Autodesk Inventor part; units mm, degrees
ref_plane "YZ Plane" through (0, 0, 0) normal (1, 0, 0) x (0, 1, 0)
ref_plane "XZ Plane" through (0, 0, 0) normal (0, 1, 0) x (-1, 0, 0)
ref_plane "XY Plane" through (0, 0, 0) normal (0, 0, 1) x (1, 0, 0)
sketch "スケッチ1" plane through (0, 0, 0) normal (1, 0, 0) x (0, 1, 0)
  circle A0 centre (0, 0) radius 4
  dimension "d0" = 8
extrude "押し出し1" add sketch "スケッチ1" along normal blind 25.5
sketch "スケッチ2" plane through (25.5, 0, 0) normal (1, 0, 0) x (0, 0, -1)
  circle A0 centre (0, 0) radius 6
  circle A1 centre (0, 0) radius 4
  dimension "d3" = 12
extrude "押し出し2" add sketch "スケッチ2" against normal blind 2.9
sketch "スケッチ3" plane through (22.6, 0, 0) normal (-1, 0, 0) x (0, 0, 1)
  circle A0 centre (0, 0) radius 3.6421
  circle A1 centre (-0.1483, 0) radius 6.8
  dimension "d6" = 13.6
extrude "押し出し3" add sketch "スケッチ3" along normal blind 2.6
sketch "スケッチ4" plane through (20, 0, -0.1483) normal (-1, 0, 0) x (0, 0, 1)
  circle A0 centre (0.1483, 0) radius 4
  circle A1 centre (0.1483, 0) radius 6
extrude "押し出し4" add sketch "スケッチ4" along normal blind 2.9
sketch "スケッチ5" plane through (25.5, 0, 0) normal (1, 0, 0) x (0, 0, -1)
  circle A0 centre (0, 0) radius 3
  dimension "d11" = 6
extrude "押し出し5" cut sketch "スケッチ5" against normal blind 1
properties part number "encoderaxis"
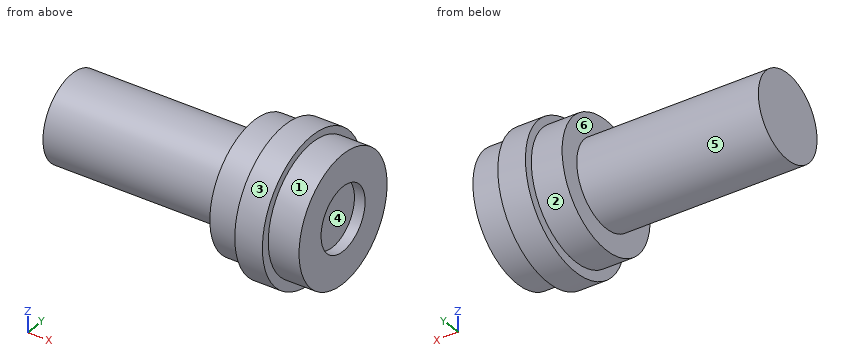
Read the model definition and answer for the solid it produces. Units are mm, in the model's axes. Face numbers are marked on the shaded views. A direction names the side the tool comes from. Give positions to 0.01 mm unless a question says otherwise; leave off trailing zeros. Write each loop counter-clockwise with the first axis right and the second up, starting at its lowest first coordinate (ties: lowest second). Pieces come first, ordered by that corner, then holes. Notation, with made-up numbers: (12.5, 8.25) - (70.5, 8.25) arc R17 cw to (70.5, 15.25) - close; hole circle Ø9 at (15, -38). An arc over 180 degrees is marked (long way). Use CSV: the item, a comma, the result in double quotes. Start each with the question number.
(1) Find section C-C (z = 0). Give the vertices of the cut face in (x, y), plus the area to 3 significant figures.
(2) Find section B-B (x = 19.5). Give the vertices of the cut face in (y, z).
(3) Determine the mould class of the marked faces 4, 5 and 6 for opening direction Y: +Y half, -Y half, draft (parallel to the pull), parting line (faces both ways), or undercut.
(4) Find section D-D (y = 5.25). Give the vertices of the cut face in (x, z).
(5) Consider line 1 along Y through (x, z) = (24.8, 0); line 2 along X through (y, z) = (-4.5, 0); line 3 along X through (y, z) = (-5, -3.5). Determine where each line is inside the solid, lowest interval first.
(6) Given P1, Ø2, axis at x = 22.5, y = -5, coming from the -Z side; P2, Ø1, axis at x = 22.5, y = 2.5, coming from the -Z side; P3, Ø1.8, axis at y = -1.5, z = 0, coming from the +X side, each flat-ended and moving along its own axis, determine where each tip first touches the part or whether it passes through.
(7) Find section A-A (y = 0). Give the vertices of the cut face in (x, z).
(8) For the marked faces 1, 2 and 3, determine the directions among +Z, -Z, +X, -X, +Y, -Y from which every point of the face is accessible in a straight line to the end or side of a thin tool.
Findings below:
1,outline,"(0, -4) - (17.1, -4) - (17.1, -6) - (20, -6) - (20, -6.8) - (22.6, -6.8) - (22.6, -6) - (25.5, -6) - (25.5, -3) - (24.5, -3) - (24.5, 3) - (25.5, 3) - (25.5, 6) - (22.6, 6) - (22.6, 6.8) - (20, 6.8) - (20, 6) - (17.1, 6) - (17.1, 4) - (0, 4) - close"
1,area,"236 mm2"
2,outline,"circle Ø12 at (0, 0)"
3,face 4,"undercut"
3,face 5,"parting line"
3,face 6,"draft"
4,outline,"(17.1, -2.9) - (20, -2.9) - (20, -4.47) - (22.6, -4.47) - (22.6, -2.9) - (25.5, -2.9) - (25.5, 2.9) - (22.6, 2.9) - (22.6, 4.17) - (20, 4.17) - (20, 2.9) - (17.1, 2.9) - close"
5,line 1,"-6 to -3, 3 to 6"
5,line 2,"17.1 to 25.5"
5,line 3,"20 to 22.6"
6,P1,"z = -5.65"
6,P2,"z = -6.65"
6,P3,"x = 24.5"
7,outline,"(0, -4) - (17.1, -4) - (17.1, -6) - (20, -6) - (20, -6.95) - (22.6, -6.95) - (22.6, -6) - (25.5, -6) - (25.5, -3) - (24.5, -3) - (24.5, 3) - (25.5, 3) - (25.5, 6) - (22.6, 6) - (22.6, 6.65) - (20, 6.65) - (20, 6) - (17.1, 6) - (17.1, 4) - (0, 4) - close"
8,face 1,"+X"
8,face 2,"-X"
8,face 3,"+X, -X"
